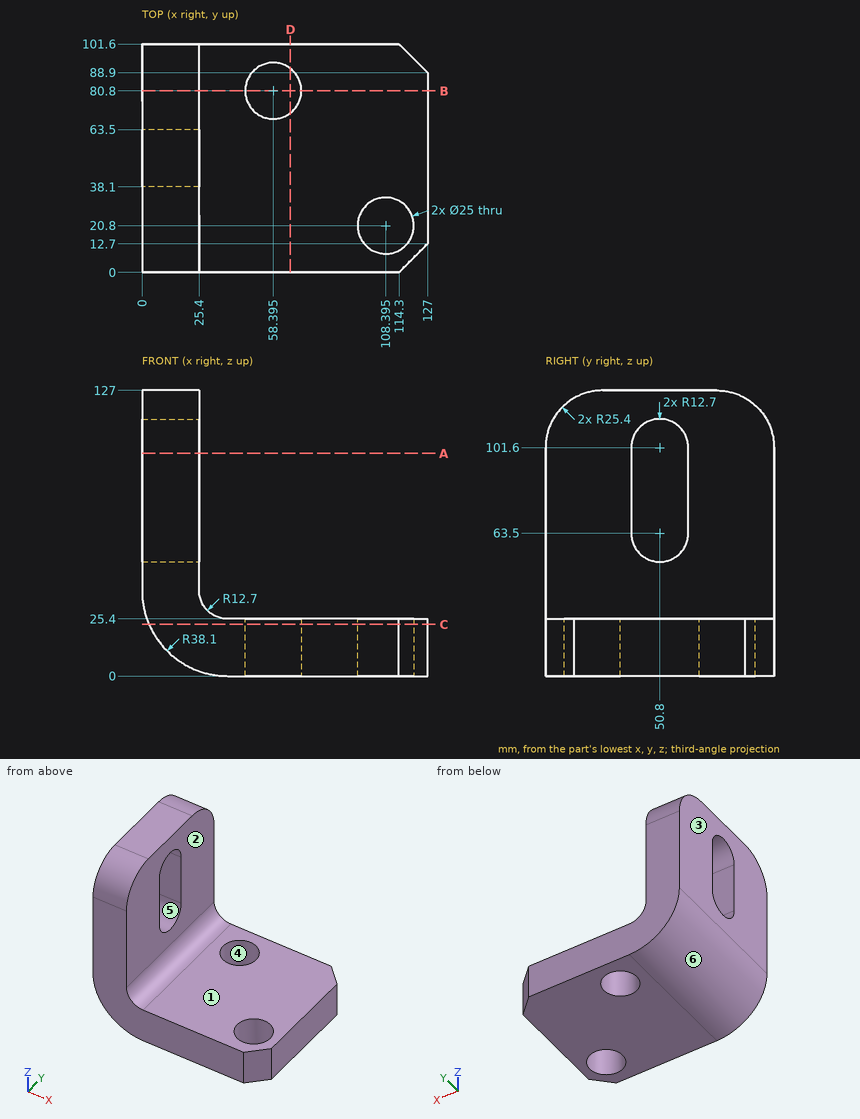
Could you check a few things on this drawing? It's one solid part, dimensions in mm from its lowest x, y, z. A direction names the side the tool comes from. Coordinates: 2 decimals unless noted, no trailing zeros. Order: outer loops, then holes, each group sorted by start corner. A loop starts at its lowest first (then second) coordinate and runs counter-clockwise, first axis right, second up. Notation, with made-up numbers: (-22.75, 74) - (2.25, 74) arc R33 ccw to (2.25, 104) - close; hole circle Ø8 at (-7.75, 75). An arc over 180 degrees is marked (long way). One line per question, with ' | ' between items.
(1) Suppose I cut it at A-A on z = 99. List the corners of the cut face in (x, y) for me, and give its area (3 significant figures).
Report:
outline: (0, 0) - (25.4, 0) - (25.4, 38.1) - (0, 38.1) - close; (0, 63.5) - (25.4, 63.5) - (25.4, 101.6) - (0, 101.6) - close | area: 1,940 mm2
(2) Will these pins go through, and if not, where does the flat tip stop? pin 1 (8 mm diameter, centred on y = 40.5, z = 54, fed in from +X); pin 2 (6 mm diameter, centred on x = 16.5, z = 113.5, fed in from -Y); pin 3 (8 mm diameter, centred on x = 89.5, y = 64.5, fed in from +Z).
Report:
pin 1: stops at x = 25.4 | pin 2: stops at y = 1.61 | pin 3: stops at z = 25.4
(3) For the marked faces 5 and 6, which set-ups out of +Z, -Z, +X, -X, +Y, -Y let a thin tool reach every point of the face, with its end or its side?
Report:
face 5: +X, -X | face 6: -Z, -X, +Y, -Y
(4) If we mould it in two halves opening along X, with no side actions, what happens to the marked faces 1, 2, 3 and 4? For each: pulls with the +X half, pulls with the -X half, needs draft (parallel to the pull), parting line crosses it, or undercut.
Report:
face 1: needs draft | face 2: pulls with the +X half | face 3: pulls with the -X half | face 4: undercut
(5) Suppose I cut it at D-D on x = 66. List the corners of the cut face in (y, z) for me, and give its area (3 significant figures).
Report:
outline: (0, 0) - (70.88, 0) - (70.88, 25.4) - (0, 25.4) - close; (90.72, 0) - (101.6, 0) - (101.6, 25.4) - (90.72, 25.4) - close | area: 2,080 mm2
(6) Suppose I cut it at C-C on z = 23. List the corners of the cut face in (x, y) for me (1 decimal).
Report:
outline: (3.1, 0) - (114.3, 0) - (127, 12.7) - (127, 88.9) - (114.3, 101.6) - (3.1, 101.6) - close; hole circle Ø25 at (58.4, 80.8); hole circle Ø25 at (108.4, 20.8)
(7) Suppose I cut it at B-B on y = 80.8. List the corners of the cut face in (x, z) for me (1 decimal).
Report:
outline: (0, 38.1) arc R38.1 ccw to (38.1, 0) - (45.9, 0) - (45.9, 25.4) - (38.1, 25.4) arc R12.7 cw to (25.4, 38.1) - (25.4, 126.6) - (0, 126.6) - close; (70.9, 0) - (127, 0) - (127, 25.4) - (70.9, 25.4) - close
(8) If I drill on L1, parallel to Y at x = 18, z = 72; L2, parallel to Z at x = 73, y = 34.5, over which ranges is the centre line in solid material (lowest first)?
Report:
L1: y = 0 to 38.1, 63.5 to 101.6 | L2: z = 0 to 25.4
